The listing builds one solid part. Answer for the finished solid, in the listing's coordinates (mm). Coordinates: 2 decimals unless noted, no trailing zeros. Loops run counter-clockwise (first coordinate to the right, second up) from the corner with the lowest first, then second, coordinate; pieces in that order, holes last. Notation, with made-up numbers: M 75,89.25 L 113,89.25 A30 cw 113,115.25 Z; hole C -16.5,10.25 d5. An arc over 180 degrees is marked long. Answer as a JSON object with one key per item and string values. Group by question number.
1. Straight lines are drawn through the part: L1, parallel to X at y = -2, z = 2.05; L2, parallel to X at y = -16, z = 2.9; L3, parallel to Z at x = -12, y = -7.5. For each, find the intervals that lie inside material, in ascending order.
2. Given pin 1 (9 mm diameter, centred on x = 27.5, y = -4, fed in from +Z); pin 2 (0.8 mm diameter, centred on x = 44, z = 3, fed in from +Y), each flat-ended and moving along its own axis, determine where each tip first touches the part or whether it passes through.
3. A cutting plane is placed at B-B on y = 5. Give the vertices of the cut face in (x, z).
4. A cutting plane is placed at C-C on y = -4.5. State how many separate pieces and enclosed holes the cut face has, and give its area (3 significant figures).
5. A cutting plane is placed at A-A on x = -12. Give the vertices of the cut face in (y, z).
from build123d import *

# Parameters (mm, degrees)
SKETCH_W        = 90
SKETCH_H        = 44
PAD_DEPTH       = 2
POCKET_DEPTH    = 1
POCKET001_DEPTH = 5
SKETCH003_W     = 12
SKETCH003_H     = 1.5
PAD001_DEPTH    = 2
SKETCH004_W     = 2
SKETCH004_H     = 44
PAD002_DEPTH    = 2.5
SKETCH005_W     = 2.5
SKETCH005_H     = 7
PAD003_DEPTH    = 3.5
SKETCH006_W     = 85
SKETCH006_H     = 1
PAD004_DEPTH    = 0.5
PAD005_DEPTH    = 0.5
POCKET002_DEPTH = 90.001


with BuildPart() as part:
    # Sketch → Pad (new body)
    with BuildSketch(Plane.XY):
        Rectangle(SKETCH_W, SKETCH_H)
    extrude(amount=PAD_DEPTH)

    # Sketch001 → Pocket (cut)
    with BuildSketch(Plane.XY.offset(2)):
        with BuildLine():
            Line((-30, 0), (-30, -13))
            Line((-30, -13), (-22, -13))
            Line((-22, -13), (-22, 0))
            ThreePointArc((-22, 0), (-26, 0.630683), (-30, 0))
        make_face()
        with BuildLine():
            Line((22, 0), (22, -13))
            Line((22, -13), (30, -13))
            Line((30, -13), (30, 0))
            ThreePointArc((30, 0), (26, 0.630683), (22, 0))
        make_face()
    extrude(amount=-POCKET_DEPTH, mode=Mode.SUBTRACT)

    # Sketch002 → Pocket001 (cut)
    with BuildSketch(Plane.XY.offset(1)):
        with BuildLine():
            Line((-29, -1), (-29, -12))
            Line((-29, -12), (-26.5, -12))
            Line((-26.5, -0.594375), (-26.5, -12))
            ThreePointArc((-26.5, -0.594375), (-27.761713, -0.724996), (-29, -1))
        make_face()
        with BuildLine():
            Line((-23, -12.000917), (-23, -1.000917))
            ThreePointArc((-23, -1.000917), (-24.238285, -0.72589), (-25.5, -0.595257))
            Line((-25.5, -0.595257), (-25.5, -12.000917))
            Line((-25.5, -12.000917), (-23, -12.000917))
        make_face()
        with BuildLine():
            Line((23, -1.000917), (23, -12.000917))
            Line((25.318595, -12.000917), (23, -12.000917))
            Line((25.318595, -0.605014), (25.318595, -12.000917))
            ThreePointArc((25.318595, -0.605014), (24.148684, -0.740808), (23, -1.000917))
        make_face()
        with BuildLine():
            Line((29, -12), (29, -1))
            ThreePointArc((29, -1), (27.761713, -0.724996), (26.5, -0.594375))
            Line((26.5, -0.594375), (26.5, -12))
            Line((26.5, -12), (29, -12))
        make_face()
    extrude(amount=-POCKET001_DEPTH, mode=Mode.SUBTRACT)

    # Sketch003 → Pad001 (new body)
    with BuildSketch(Plane.XY.offset(2)):
        with Locations((-26, -13.75)):
            Rectangle(SKETCH003_W, SKETCH003_H)
        with Locations((26, -13.75)):
            Rectangle(SKETCH003_W, SKETCH003_H)
    extrude(amount=PAD001_DEPTH)

    # Sketch004 → Pad002 (new body)
    with BuildSketch(Plane(origin=(0, 0, 0), x_dir=(1, 0, 0), z_dir=(0, 0, -1))):
        with Locations((-44, 0)):
            Rectangle(SKETCH004_W, SKETCH004_H)
        with Locations((44, 0)):
            Rectangle(SKETCH004_W, SKETCH004_H)
    extrude(amount=-PAD002_DEPTH)

    # Sketch005 → Pad003 (new body)
    with BuildSketch(Plane(origin=(0, 0, 0), x_dir=(1, 0, 0), z_dir=(0, 0, -1))):
        with Locations((-43.75, 18.5)):
            Rectangle(SKETCH005_W, SKETCH005_H)
        with Locations((43.75, 18.5)):
            Rectangle(SKETCH005_W, SKETCH005_H)
    extrude(amount=-PAD003_DEPTH)

    # Sketch006 → Pad004 (new body)
    with BuildSketch(Plane.XY.offset(2)):
        with Locations((0, -16.5)):
            Rectangle(SKETCH006_W, SKETCH006_H)
    extrude(amount=PAD004_DEPTH)

    # Sketch007 → Pad005 (new body)
    with BuildSketch(Plane.XY.offset(2)):
        with BuildLine():
            Line((-30.75, -13), (-30.75, 1.152062))
            Line((-30.75, 1.152062), (-29.75, 1.152062))
            ThreePointArc((-22.25, 1.152062), (-26, 1.753049), (-29.75, 1.152062))
            Line((-22.25, 1.152062), (-21.25, 1.152062))
            Line((-21.25, 1.152062), (-21.25, -13))
            Line((-21.25, -13), (-22, -13))
            Line((-22, -13), (-22, 0))
            ThreePointArc((-22, 0), (-26, 0.753049), (-30, 0))
            Line((-30, -13), (-30, 0))
            Line((-30, -13), (-30.75, -13))
        make_face()
        with BuildLine():
            Line((21.25, 1.152062), (21.25, -13))
            Line((21.25, -13), (22, -13))
            Line((22, -13), (22, 0))
            ThreePointArc((30, 0), (26, 0.753049), (22, 0))
            Line((30, 0), (30, -13))
            Line((30, -13), (30.75, -13))
            Line((30.75, -13), (30.75, 1.152062))
            Line((30.75, 1.152062), (29.75, 1.152062))
            ThreePointArc((29.75, 1.152062), (26, 1.753049), (22.25, 1.152062))
            Line((21.25, 1.152062), (22.25, 1.152062))
        make_face()
    extrude(amount=PAD005_DEPTH)

    # Sketch008 → Pocket002 (cut, through all)
    with BuildSketch(Plane(origin=(-45, 0, 0), x_dir=(0, -1, 0), z_dir=(-1, 0, 0))):
        Polygon((-25.209874, 17.987658), (-5.209874, 17.987658), (-25.209874, -7.012342), align=None)
    extrude(amount=-POCKET002_DEPTH, mode=Mode.SUBTRACT)


solid = part.part
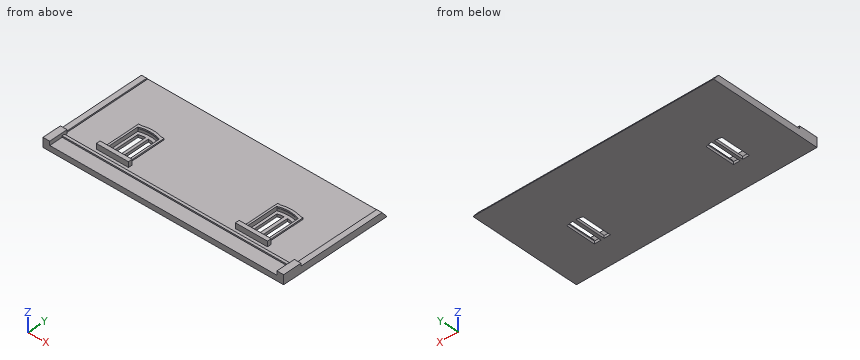
From the geometry:
{
 "1": {"L1": "x = -45 to -43, -30.75 to -30, -22 to -21.25, 21.25 to 22, 30 to 30.75, 43 to 45", "L2": "x = -45 to -42.5, 42.5 to 45", "L3": "z = 0 to 2"},
 "2": {"pin 1": "stops at z = 2.5", "pin 2": "stops at y = -15"},
 "3": {"outline": "M -45,0 L 45,0 L 45,2.5 L 43,2.5 L 43,2 L -43,2 L -43,2.5 L -45,2.5 Z"},
 "4": {"separate pieces": "5", "enclosed holes": "0", "area": "158 mm²"},
 "5": {"outline": "M -22,0 L 19.6,0 L 18,2 L -16,2 L -16,2.5 L -17,2.5 L -17,2 L -22,2 Z"}
}
